For this review, take the finished solid that the model builds, in its own axes (mm). Face numbers are marked on the shaded views. A direction names the side the tool comes from. Coordinates: 2 decimals unless noted, no trailing zeros. Loops run counter-clockwise (first coordinate to the right, second up) from the corner with the lowest first, then second, coordinate; pieces in that order, holes last. Notation, with made-up numbers: (-32, -3.5) -> (-12, -3.5) arc R19 ccw to (-12, 24.5) -> close; hole circle Ø11 at (4.25, -19). An arc over 180 degrees is marked (long way). One line per item, written item: value.
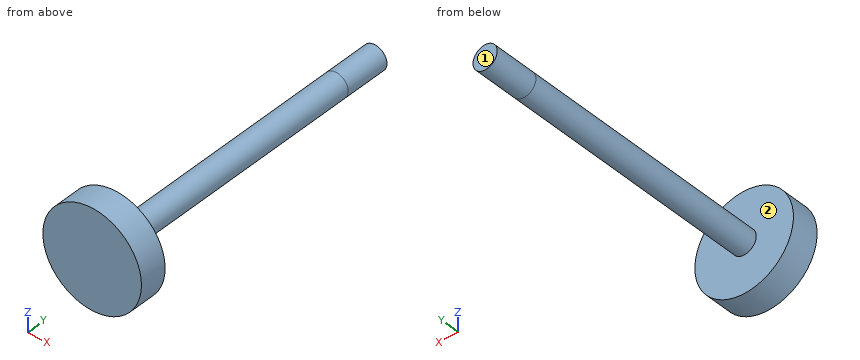
Autodesk Inventor part; units mm, degrees
ref_plane "YZ Plane" through (0, 0, 0) normal (1, 0, 0) x (0, 1, 0)
ref_plane "XZ Plane" through (0, 0, 0) normal (0, 1, 0) x (-1, 0, 0)
ref_plane "XY Plane" through (0, 0, 0) normal (0, 0, 1) x (1, 0, 0)
sketch "Boceto1" plane through (0, 0, 0) normal (0, 1, 0) x (-1, 0, 0)
  circle A0 centre (0, 0) radius 1.45
  dimension "d0" = 2.9
extrude "Extrusión1" add sketch "Boceto1" against normal blind 30.7
sketch "Boceto2" plane through (0, -30.7, 0) normal (0, -1, 0) x (1, 0, 0)
  circle A0 centre (0, 0) radius 5.9
  dimension "d3" = 11.8
extrude "Extrusión2" add sketch "Boceto2" along normal blind 3.3
sketch "Boceto3" plane through (0, 0, 0) normal (0, 1, 0) x (1, 0, 0)
  circle A0 centre (0, 0) radius 1.45
  circle A1 centre (0, 0) radius 1.45
  dimension "d6" = 2.9
extrude "Extrusión3" add sketch "Boceto3" along normal blind 5.4
properties part number "Embolo" material "Aluminio 6061"
1. Take a section at C-C, the plane y = -5. Give the boundary of the cut face in (x, z).
Return value:
outline: circle Ø2.9 at (0, 0)
2. Take a section at B-B, the plane z = 0. Give the boundary of the cut face in (x, y).
Return value:
outline: (-5.9, -34) -> (5.9, -34) -> (5.9, -30.7) -> (1.45, -30.7) -> (1.45, 5.4) -> (-1.45, 5.4) -> (-1.45, -30.7) -> (-5.9, -30.7) -> close
3. Insertion check: pin 1 Ø1 at (y, z) = (-26, 0) entering from +X; pin 2 Ø1.5 at (x, y) = (1.5, -5.5) entering from +Z; pin 3 Ø1.5 at (y, z) = (1, -1.5) entering from -X. Each pin has a flat end and moves straight along its axis. Give the tip position at first contact, or say it passes through.
Return value:
pin 1: stops at x = 1.45
pin 2: stops at z = 1.24
pin 3: stops at x = -1.24
4. For the marked faces 1 and 2, list the 3-axis set-ups (+Z, -Z, +X, -X, +Y, -Y) from which the entire face can be reached by the end or side of a thin tool; tool diameter is ignored.
Return value:
face 1: +Z, -Z, +X, -X, +Y
face 2: +Y
5. Take a section at D-D, the plane z = 5. Give the boundary of the cut face in (x, y).
Return value:
outline: (-3.13, -34) -> (3.13, -34) -> (3.13, -30.7) -> (-3.13, -30.7) -> close
6. Take a section at A-A, the plane x = 0. Give the boundary of the cut face in (y, z).
Return value:
outline: (-34, -5.9) -> (-30.7, -5.9) -> (-30.7, -1.45) -> (5.4, -1.45) -> (5.4, 1.45) -> (-30.7, 1.45) -> (-30.7, 5.9) -> (-34, 5.9) -> close
7. To check wall thickness, follow probe 1 along Y at (x, z) = (2.75, -0.75); probe 2 along X at (y, z) = (-30, 0); probe 3 along X at (y, z) = (-20, 1.25). State the ranges of each line that lie inside material, in increasing order. Write a range as from..to.
Return value:
probe 1: y = -34..-30.7
probe 2: x = -1.45..1.45
probe 3: x = -0.73..0.73
